Design review of the part built by this model. Coordinates are the model's own, in mm. Round coordinates to 2 decimals unless told otherwise and drop trailing zeros. Use CSV: the item, a comma, the result in double quotes. Start each with the question number.
from build123d import *

# Parameters (mm, degrees)
BASEEXTRUDE_DEPTH   = 3.175
SKETCH6_R           = 1.5
MAINMOUNTCUT_DEPTH  = 3.175
SKETCH7_R           = 1.6
SKETCH7_W           = 50.8
SKETCH7_H           = 6.35
WALLCUT_DEPTH       = 4.175
SKETCH8_W           = 38.1
SKETCH8_H           = 3.175
WIREMOUNTCUT_DEPTH  = 4.175
SKETCH9_R           = 1.6
CUT_EXTRUDE3_DEPTH  = 4.175
SKETCH11_W          = 6.35
SKETCH11_H          = 50.8
CUT_EXTRUDE4_DEPTH  = 4.175
SKETCH14_W          = 6.35
SKETCH14_H          = 15.24
CUT_EXTRUDE6_DEPTH  = 4.175
SKETCH15_R          = 1.190625
CUT_EXTRUDE7_DEPTH  = 4.175
SKETCH16_R          = 1.190625
CUT_EXTRUDE8_DEPTH  = 4.175
SKETCH17_W          = 76.2
SKETCH17_H          = 91.44
SKETCH17_W_2        = 64.77
CUT_EXTRUDE9_DEPTH  = 4.175
SKETCH18_R          = 1.6
SKETCH18_W          = 25.4
SKETCH18_H          = 6.35
CUT_EXTRUDE10_DEPTH = 4.175


with BuildPart() as part:
    # Sketch3 → BaseExtrude (new body)
    with BuildSketch(Plane(origin=(0, 0, 0), x_dir=(1, 0, 0), z_dir=(0, 1, 0))):
        with BuildLine():
            Line((-156.21, -88.9), (156.21, -88.9))
            ThreePointArc((156.21, -88.9), (174.170512242, -81.460512242), (181.61, -63.5))
            Line((181.61, -63.5), (181.61, 63.5))
            ThreePointArc((181.61, 63.5), (174.170512242, 81.460512242), (156.21, 88.9))
            Line((156.21, 88.9), (-156.21, 88.9))
            ThreePointArc((-156.21, 88.9), (-174.170512242, 81.460512242), (-181.61, 63.5))
            Line((-181.61, 63.5), (-181.61, -63.5))
            ThreePointArc((-181.61, -63.5), (-174.170512242, -81.460512242), (-156.21, -88.9))
        make_face()
    extrude(amount=-BASEEXTRUDE_DEPTH)

    # Sketch6 → MainMountCut (cut)
    with BuildSketch(Plane(origin=(0, 0, 0), x_dir=(1, 0, 0), z_dir=(0, 1, 0))):
        with Locations((-157.988, 15.875)):
            Circle(SKETCH6_R)
        with Locations((-157.988, -15.875)):
            Circle(SKETCH6_R)
        with Locations((165.862, -15.875)):
            Circle(SKETCH6_R)
        with Locations((165.862, 15.875)):
            Circle(SKETCH6_R)
    extrude(amount=-MAINMOUNTCUT_DEPTH, mode=Mode.SUBTRACT)

    # Sketch7 → WallCut (cut, through all)
    with BuildSketch(Plane(origin=(0, 0, 0), x_dir=(1, 0, 0), z_dir=(0, 1, 0))):
        with Locations((51.223333333, 79.375)):
            Circle(SKETCH7_R)
        with Locations((-50.376666667, 79.375)):
            Circle(SKETCH7_R)
        with Locations((-50.376666667, -79.375)):
            Circle(SKETCH7_R)
        with Locations((51.223333333, -79.375)):
            Circle(SKETCH7_R)
        with Locations((102.023333333, -79.375)):
            Rectangle(SKETCH7_W, SKETCH7_H)
        with Locations((0.423333333, -79.375)):
            Rectangle(SKETCH7_W, SKETCH7_H)
        with Locations((-101.176666667, -79.375)):
            Rectangle(SKETCH7_W, SKETCH7_H)
        with Locations((102.023333333, 79.375)):
            Rectangle(SKETCH7_W, SKETCH7_H)
        with Locations((0.423333333, 79.375)):
            Rectangle(SKETCH7_W, SKETCH7_H)
        with Locations((-101.176666667, 79.375)):
            Rectangle(SKETCH7_W, SKETCH7_H)
    extrude(amount=-WALLCUT_DEPTH, mode=Mode.SUBTRACT)

    # Sketch8 → WireMountCut (cut, through all)
    with BuildSketch(Plane(origin=(0, 0, 0), x_dir=(1, 0, 0), z_dir=(0, 1, 0))):
        with Locations((124.46, -59.69)):
            Rectangle(SKETCH8_W, SKETCH8_H)
        with Locations((124.46, -29.845)):
            Rectangle(SKETCH8_W, SKETCH8_H)
        with Locations((124.46, 0)):
            Rectangle(SKETCH8_W, SKETCH8_H)
        with Locations((124.46, 29.845)):
            Rectangle(SKETCH8_W, SKETCH8_H)
        with Locations((124.46, 59.69)):
            Rectangle(SKETCH8_W, SKETCH8_H)
    extrude(amount=-WIREMOUNTCUT_DEPTH, mode=Mode.SUBTRACT)

    # Sketch9 → Cut-Extrude3 (cut, through all)
    with BuildSketch(Plane(origin=(0, 0, 0), x_dir=(1, 0, 0), z_dir=(0, 1, 0))):
        with Locations((118.11, 50.8)):
            Circle(SKETCH9_R)
        with Locations((118.11, -50.8)):
            Circle(SKETCH9_R)
        with Locations((-149.86, -50.8)):
            Circle(SKETCH9_R)
        with Locations((-149.86, 50.8)):
            Circle(SKETCH9_R)
    extrude(amount=-CUT_EXTRUDE3_DEPTH, mode=Mode.SUBTRACT)

    # Sketch11 → Cut-Extrude4 (cut, through all)
    with BuildSketch(Plane(origin=(0, 0, 0), x_dir=(1, 0, 0), z_dir=(0, 1, 0))):
        with Locations((-18.415, 0)):
            Rectangle(SKETCH11_W, SKETCH11_H)
    extrude(amount=-CUT_EXTRUDE4_DEPTH, mode=Mode.SUBTRACT)

    # Sketch14 → Cut-Extrude6 (cut, through all)
    with BuildSketch(Plane(origin=(0, 0, 0), x_dir=(1, 0, 0), z_dir=(0, 1, 0))):
        with Locations((-141.156855902, -44.45)):
            Rectangle(SKETCH14_W, SKETCH14_H)
    extrude(amount=-CUT_EXTRUDE6_DEPTH, mode=Mode.SUBTRACT)

    # Sketch15 → Cut-Extrude7 (cut, through all)
    with BuildSketch(Plane(origin=(0, 0, 0), x_dir=(1, 0, 0), z_dir=(0, 1, 0))):
        with Locations((67.31, -58.42)):
            Circle(SKETCH15_R)
        with Locations((-49.53, -58.42)):
            Circle(SKETCH15_R)
        with Locations((-49.53, 58.42)):
            Circle(SKETCH15_R)
        with Locations((67.31, 58.42)):
            Circle(SKETCH15_R)
        with Locations((137.16, -38.1)):
            Circle(SKETCH15_R)
        with Locations((118.11, -38.1)):
            Circle(SKETCH15_R)
        with Locations((137.16, 38.1)):
            Circle(SKETCH15_R)
        with Locations((118.11, 38.1)):
            Circle(SKETCH15_R)
    extrude(amount=-CUT_EXTRUDE7_DEPTH, mode=Mode.SUBTRACT)

    # Sketch16 → Cut-Extrude8 (cut, through all)
    with BuildSketch(Plane(origin=(0, 0, 0), x_dir=(1, 0, 0), z_dir=(0, 1, 0))):
        with Locations((-130.81, -28.5)):
            Circle(SKETCH16_R)
        with Locations((-130.81, 28.5)):
            Circle(SKETCH16_R)
    extrude(amount=-CUT_EXTRUDE8_DEPTH, mode=Mode.SUBTRACT)

    # Sketch17 → Cut-Extrude9 (cut, through all)
    with BuildSketch(Plane(origin=(0, 0, 0), x_dir=(1, 0, 0), z_dir=(0, 1, 0))):
        with Locations((41.91, 0)):
            Rectangle(SKETCH17_W, SKETCH17_H)
        with Locations((-73.025, 0)):
            Rectangle(SKETCH17_W_2, SKETCH17_H)
    extrude(amount=-CUT_EXTRUDE9_DEPTH, mode=Mode.SUBTRACT)

    # Sketch18 → Cut-Extrude10 (cut, through all)
    with BuildSketch(Plane(origin=(0, 0, 0), x_dir=(1, 0, 0), z_dir=(0, 1, 0))):
        with Locations((-8.636, -66.675)):
            Circle(SKETCH18_R)
        with Locations((-8.636, 66.675)):
            Circle(SKETCH18_R)
        with Locations((10.414, -66.675)):
            Rectangle(SKETCH18_W, SKETCH18_H)
        with Locations((10.414, 66.675)):
            Rectangle(SKETCH18_W, SKETCH18_H)
    extrude(amount=-CUT_EXTRUDE10_DEPTH, mode=Mode.SUBTRACT)


solid = part.part
Q1. Take a section at A-A (y = -1.1). Give the number of separate pieces and of enclosed holes in the cut face, plus the area to 3 significant figures.
Q2. Clearance check with flat-ended pins moving along their axes: pin 1 (2.5 mm diameter, centred on x = 165.862, z = 15.875, fed in from +Y); pin 2 (1.6 mm diameter, centred on y = -1.5, z = -67, fed in from -X); pin 3 (1 mm diameter, centred on y = -1, z = -79.5, fed in from +X). State where each tip first meets the part, or that it passes through.
Q3. For L1, parallel to X at y = -2.65, z = -35; L2, parallel to Z at x = -149.86, y = -0.85; L3, parallel to X at y = -3, z = 50.5, list the stretches that pass through material, from the lowest coordinate up. Write a range as [from, to].
Findings below:
1,separate pieces,"1"
1,enclosed holes,"41"
1,area,"47,700 mm^2"
2,pin 1,"passes through"
2,pin 2,"stops at x = -181.47"
2,pin 3,"stops at x = 176.33"
3,L1,"x = [-181.61, -105.41], [-40.64, 3.81], [80.01, 181.61]"
3,L2,"z = [-88.9, -52.4], [-49.2, 49.2], [52.4, 88.9]"
3,L3,"x = [-181.61, -151.43], [-148.29, -144.33], [-137.98, 116.54], [119.68, 181.61]"
